from build123d import *

# Parameters (mm, degrees)
F0_W     = 38.1
F0_H     = 6.35
F1_DEPTH = 25.4
F3_DEPTH = 25.4
F4_W     = 12.7
F4_H     = 6.35
F5_DEPTH = 25.401
F6_W     = 6.35
F6_H     = 12.7
F7_DEPTH = 19.051


with BuildPart() as f1:
    # F0 (on Right) → F1 (new body)
    with BuildSketch(Plane.YZ):
        with Locations((-19.05, 3.175)):
            Rectangle(F0_W, F0_H)
    extrude(amount=F1_DEPTH)

    # F2 (on Front) → F3 (join)
    with BuildSketch(Plane.XZ):
        Polygon((0, 25.4), (0, 6.35), (25.4, 6.35), align=None)
    extrude(amount=F3_DEPTH)

    # F4 (on Right) → F5 (cut, through all)
    with BuildSketch(Plane.YZ):
        with Locations((-19.05, 22.225)):
            Rectangle(F4_W, F4_H)
    extrude(amount=F5_DEPTH, mode=Mode.SUBTRACT)

    # F6 (on face) → F7 (cut, through all)
    with BuildSketch(Plane.XY.offset(6.35)):
        with Locations((22.225, -19.05)):
            Rectangle(F6_W, F6_H)
    extrude(amount=F7_DEPTH, mode=Mode.SUBTRACT)


solid = f1.part
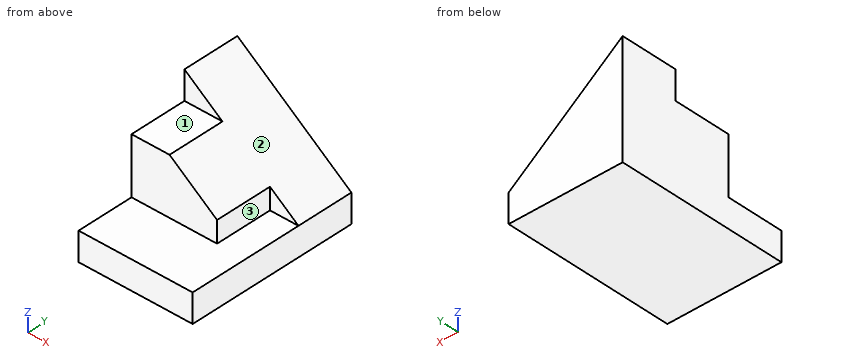
Verification items for the finished model (mm, model axes). Face numbers are marked on the shaded views. A direction names the side the tool comes from. Give positions to 0.01 mm unless a question says otherwise; leave off trailing zeros. Loops run counter-clockwise (first coordinate to the right, second up) from the corner with the lowest first, then second, coordinate; pieces in that order, holes last. Notation, with made-up numbers: (-9, 44.5) - (41, 44.5) arc R10 cw to (41, 59.5) - close; hole circle Ø5 at (83, 49). An arc over 180 degrees is marked (long way). Write item = value, one per line. Start each with the question number.
Q1. Cross-section at C-C, the plane z = 7.25. Enter the section's corners in (x, y), and give its area (3 significant figures).
Q2. Cross-section at D-D, the plane x = 6. Enter the section's corners in (y, z).
Q3. Cross-section at A-A, the plane x = 3. Enter the section's corners in (y, z).
Q4. Thickness scan on line 1 (Y direction, x = 23.75, z = 6.75); line 2 (X direction, y = -24, z = 9); line 3 (Z direction, x = 21.5, y = -20). Record the ranges inside material, lowest first.
Q5. Tool access check on the marked faces 1, 2 and 3. Record the directions out of +Z, -Z, +X, -X, +Y, -Y that give a thin tool (end or side, any length) a straight path to the whole face; none if there is none.
Q6. Cross-section at B-B, the plane y = -19. Enter the section's corners in (x, z), and give its area (3 significant figures).
Q7. Depth check by flat-ended pin: P1, Ø5, axis at y = -16, z = 10, coming from the +X side; P2, Ø10, axis at x = 13.5, z = 12.5, coming from the -Y side; P3, Ø6, axis at x = 18, y = -12, coming from the -Z side; P4, Ø4, axis at x = 2.5, y = -16.5, coming from the +Z side. Enter the tip coordinate at first touch or a pass-through.
Answer key:
q1.outline = (0, -25.4) - (19.05, -25.4) - (19.05, -12.7) - (24.2, -12.7) - (24.2, 0) - (0, 0) - close
q1.area = 549 mm^2
q2.outline = (-38.1, 0) - (0, 0) - (0, 20.9) - (-12.7, 20.9) - (-12.7, 19.05) - (-25.4, 19.05) - (-25.4, 6.35) - (-38.1, 6.35) - close
q3.outline = (-38.1, 0) - (0, 0) - (0, 23.15) - (-12.7, 23.15) - (-12.7, 19.05) - (-25.4, 19.05) - (-25.4, 6.35) - (-38.1, 6.35) - close
q4.line_1 = -12.7 to 0
q4.line_2 = 0 to 19.05
q4.line_3 = 0 to 6.35
q5.face_1 = +Z, +X, -X, -Y
q5.face_2 = +Z, +X, +Y, -Y
q5.face_3 = +Z, +X, -Y
q6.outline = (0, 0) - (25.4, 0) - (25.4, 6.35) - (19.05, 6.35) - (19.05, 11.11) - (8.47, 19.05) - (0, 19.05) - close
q6.area = 361 mm^2
q7.P1 = 19.05
q7.P2 = -25.4
q7.P3 = 0
q7.P4 = 19.05
